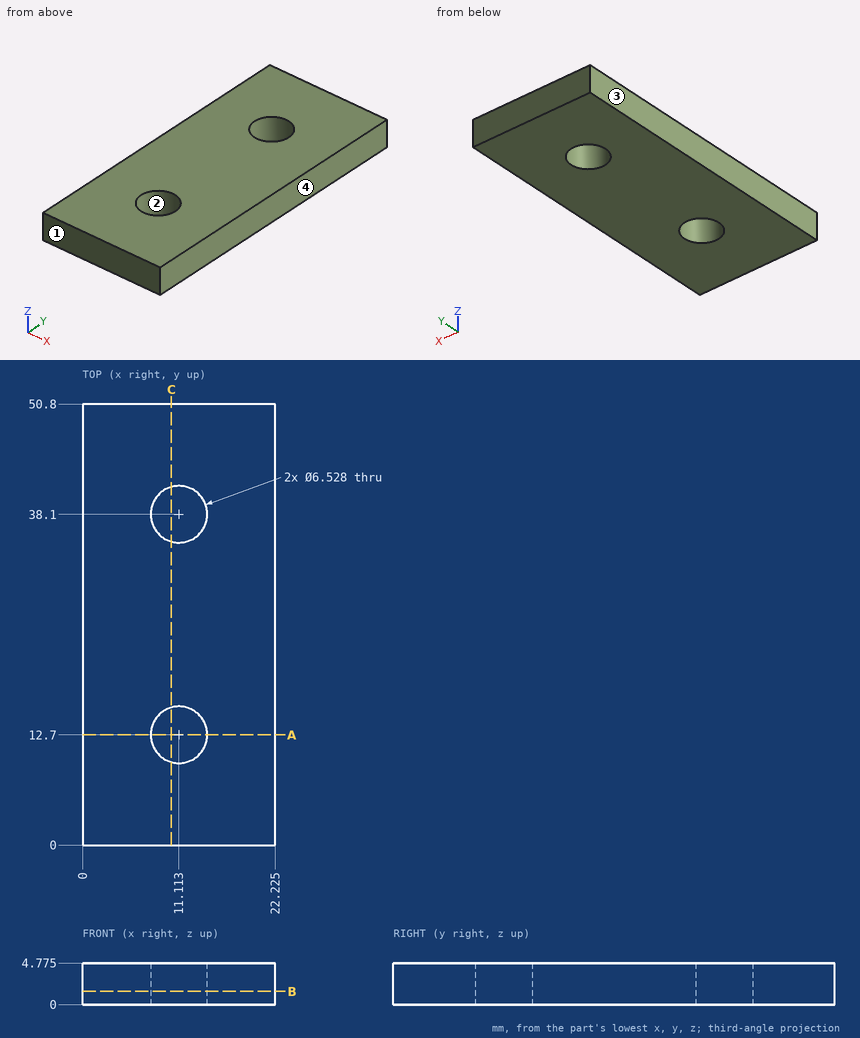
For this review, use the dimensioned drawing (mm, ordinates from the lowest corner) and the shaded views. Round coordinates to 2 decimals unless told otherwise and drop trailing zeros. Write each loop counter-clockwise with the first axis right and the second up, starting at its lowest first coordinate (ties: lowest second). Pieces come first, ordered by that corner, then holes. Notation, with made-up numbers: (19.5, 10) - (39.5, 10) arc R4 cw to (39.5, 14) - close; hole circle Ø4 at (-34, 45). An arc over 180 degrees is marked (long way). One line per item, written item: value. Start each with the question number.
1. Clearance check with flat-ended pins moving along their axes: P1, Ø4, axis at x = 11.11, y = 12.7, coming from the +Z side; P2, Ø7.5, axis at x = 11.11, y = 38.1, coming from the +Z side (1 decimal). State where each tip first meets the part, or that it passes through.
2. Consider section A-A on y = 12.7. Write out the cut boundary in (x, z) (1 decimal).
3. Consider section C-C on x = 10.25. Write out the cut boundary in (y, z) (1 decimal).
4. To check wall thickness, follow L1, parallel to Y at x = 14, z = 2.4 (1 decimal); L2, parallel to Y at x = 13.5, z = 1.55 (1 decimal); L3, parallel to X at y = 12, z = 2.95 (1 decimal). State the ranges of each line that lie inside material, in increasing order. Write a range as from..to.
5. Consider section B-B on z = 1.5. Write out the cut boundary in (x, y) (1 decimal), and give its area (3 significant figures).
6. The part is to be moulded in two halves that separate along X. For the marked faces 1, 2, 3 and 4, say which applies: released by +X, released by -X, zero draft, split by the parting line, or undercut.
Checks:
1. P1: passes through
1. P2: stops at z = 4.8
2. outline: (0, 0) - (7.8, 0) - (7.8, 4.8) - (0, 4.8) - close; (14.4, 0) - (22.2, 0) - (22.2, 4.8) - (14.4, 4.8) - close
3. outline: (0, 0) - (9.6, 0) - (9.6, 4.8) - (0, 4.8) - close; (15.8, 0) - (35, 0) - (35, 4.8) - (15.8, 4.8) - close; (41.2, 0) - (50.8, 0) - (50.8, 4.8) - (41.2, 4.8) - close
4. L1: y = 0..11.2, 14.2..36.6, 39.6..50.8
4. L2: y = 0..10.5, 14.9..35.9, 40.3..50.8
4. L3: x = 0..7.9, 14.3..22.2
5. outline: (0, 0) - (22.2, 0) - (22.2, 50.8) - (0, 50.8) - close; hole circle Ø6.5 at (11.1, 12.7); hole circle Ø6.5 at (11.1, 38.1)
5. area: 1,060 mm^2
6. face 1: zero draft
6. face 2: undercut
6. face 3: released by -X
6. face 4: released by +X
